from build123d import *

# Parameters (mm, degrees)
ESBO_O1_W                = 22.5
ESBO_O1_H                = 20.7
RESSALTO_EXTRUS_O1_DEPTH = 0.8
ESBO_O2_R                = 0.5
ESBO_O2_R_2              = 0.65
ESBO_O2_R_3              = 0.45
ESBO_O2_R_4              = 0.507049464
ESBO_O2_R_5              = 0.6
ESBO_O2_R_6              = 0.375708805
ESBO_O2_R_7              = 0.378805018
ESBO_O2_R_8              = 0.350015613
ESBO_O2_R_9              = 0.522974081
CORTE_EXTRUS_O1_DEPTH    = 2


with BuildPart() as part:
    # Esboço1 → Ressalto-extrusão1 (new body)
    with BuildSketch(Plane(origin=(0, 0, 0), x_dir=(1, 0, 0), z_dir=(0, 1, 0))):
        Rectangle(ESBO_O1_W, ESBO_O1_H)
    extrude(amount=RESSALTO_EXTRUS_O1_DEPTH)

    # Esboço2 → Corte-extrusão1 (cut)
    with BuildSketch(Plane(origin=(0, 0.8, 0), x_dir=(1, 0, 0), z_dir=(0, 1, 0))):
        with Locations(Location((-1.362497423, 4.13217589, 0), (0, 0, 270))):
            Circle(ESBO_O2_R)
        with Locations(Location((9.781964431, 1.510174659, 0), (0, 0, 270))):
            Circle(ESBO_O2_R)
        with Locations(Location((9.781964431, -3.684410863, 0), (0, 0, 270))):
            Circle(ESBO_O2_R)
        with Locations(Location((9.781964431, -6.220381714, 0), (0, 0, 270))):
            Circle(ESBO_O2_R)
        with Locations(Location((10.140573187, -9.276881362, 0), (0, 0, 270))):
            Circle(ESBO_O2_R_2)
        with Locations(Location((1.456478245, -9.018440966, 0), (0, 0, 270))):
            Circle(ESBO_O2_R_2)
        with Locations(Location((-5.049050046, 7.684323928, 0), (0, 0, 270))):
            Circle(ESBO_O2_R)
        with Locations(Location((-2.429917945, 7.684323928, 0), (0, 0, 270))):
            Circle(ESBO_O2_R)
        with Locations(Location((-1.362497423, -6.113976729, 0), (0, 0, 270))):
            Circle(ESBO_O2_R_3)
        with Locations(Location((9.868300548, 3.960954596, 0), (0, 0, 270))):
            Circle(ESBO_O2_R)
        with Locations(Location((-1.362497423, 1.510174659, 0), (0, 0, 270))):
            Circle(ESBO_O2_R_3)
        with Locations(Location((-1.362497423, -1.018750271, 0), (0, 0, 270))):
            Circle(ESBO_O2_R_3)
        with Locations(Location((2.009813707, 8.41282711, 0), (0, 0, 270))):
            Circle(ESBO_O2_R_2)
        with Locations(Location((4.713446832, 8.41282711, 0), (0, 0, 270))):
            Circle(ESBO_O2_R_2)
        with Locations(Location((7.464512117, 8.41282711, 0), (0, 0, 270))):
            Circle(ESBO_O2_R_2)
        with Locations(Location((-7.40057526, 6.840223885, 0), (0, 0, 270))):
            Circle(ESBO_O2_R_4)
        with Locations(Location((-9.173194548, -9.276881362, 0), (0, 0, 270))):
            Circle(ESBO_O2_R_5)
        with Locations(Location((-4.945655629, -9.276881362, 0), (0, 0, 270))):
            Circle(ESBO_O2_R_5)
        with Locations(Location((-9.677939464, 3.896952444, 0), (0, 0, 270))):
            Circle(ESBO_O2_R_6)
        with Locations(Location((-4.441443384, 2.017609351, 0), (0, 0, 270))):
            Circle(ESBO_O2_R_7)
        with Locations(Location((8.485674085, -1.384098552, 0), (0, 0, 270))):
            Circle(ESBO_O2_R_8)
        with Locations(Location((-10.473206437, 6.840223885, 0), (0, 0, 270))):
            Circle(ESBO_O2_R_9)
    extrude(amount=-CORTE_EXTRUS_O1_DEPTH, mode=Mode.SUBTRACT)


solid = part.part
Check sheet for the modelled part. Datum: model origin and axes. Units: mm. Give positions to 0.01 mm unless a question says otherwise; leave off trailing zeros. Write each loop counter-clockwise with the first axis right and the second up, starting at its lowest first coordinate (ties: lowest second). Pieces come first, ordered by that corner, then holes. Notation, with made-up numbers: (85.5, 62) -> (102.5, 62) arc R26 ccw to (102.5, 84) -> close; hole circle Ø1 at (41, 75.25). An arc over 180 degrees is marked (long way). One line per item, written item: value. Start each with the question number.
Item 1: Section check A-A on x = 7.75. Record the cut outline in (y, z).
Item 2: Material ranges on probe 1 along Z at (x, y) = (-5, 0.5); probe 2 along Z at (x, y) = (-2.5, 0.15); probe 3 along Z at (x, y) = (5, 0.15), recorded low to high. Write a range as from..to.
Item 3: Section check B-B on y = 0.2. State how many separate pieces and enclosed holes the cut face has, then the cut area to 4 significant figures.
Item 4: Draft check along X on faces 1 (the cylindrical face through (-5.48, 0.41, 9.55)), 2 (the flat face through (0, 0.8, 0)), 3 (the cylindrical face through (1.49, 0.41, 8.37)). Enter one of: +X half, -X half, draft (parallel to the pull), parting line (faces both ways), or undercut.
Item 5: Gauge pin test, flat end, axial feed: pin 1 (1 mm diameter, centred on x = -4.95, z = 9.28, fed in from -Y). Record the tip position at first contact, or that the pin passes through.
Results list:
1. outline: (0, -10.35) -> (0.8, -10.35) -> (0.8, -9) -> (0, -9) -> close; (0, -7.83) -> (0.8, -7.83) -> (0.8, 10.35) -> (0, 10.35) -> close
2. probe 1: -10.35..-8.18, -7.19..8.68, 9.87..10.35
2. probe 2: -10.35..-8.18, -7.19..10.35
2. probe 3: -10.35..-9, -7.83..10.35
3. separate pieces: 1
3. enclosed holes: 22
3. area: 446.5 mm²
4. face 1: undercut
4. face 2: draft
4. face 3: undercut
5. pin 1: through
